Geometry: final body of the model. Coordinates: model frame, mm. Face numbers are marked on the shaded views. A direction names the side the tool comes from. Give positions to 0.01 mm unless a question says otherwise; leave off trailing zeros. Order: outer loops, then holes, each group sorted by start corner. A loop starts at its lowest first (then second) coordinate and runs counter-clockwise, first axis right, second up. Notation, with made-up numbers: (51, 79) -> (103, 79) arc R28 ccw to (103, 111) -> close; hole circle Ø4 at (-16.75, 45). An arc over 180 degrees is marked (long way). Answer in a Markdown table with one row per item. Add a question column.
Q1. Pull-direction query (Y, two-part tool) for the marked faces 1, 2 and 3; classes: +Y half, -Y half, draft (parallel to the pull), parting line (faces both ways), or undercut.
Q2. Contact query for flat-ended pins moving along their axis: P1, Ø6, axis at x = 14.5, z = 2, coming from the +Y side; P2, Ø1, axis at x = -7.5, y = 16, coming from the -Z side; P3, Ø10, axis at x = -19, z = -1.5, coming from the +Y side. Output: stop coordinate, or through.
Q3. Cut plane C-C on x = -10.5. Return the cut outline in (y, z).
Q4. Cut plane B-B on x = 0. Return the cut outline in (y, z), and give its area (3 significant figures).
Q5. Cut plane A-A on z = -10.5. Return the cut outline in (x, y).
Q6. Set-up query: the marked faces 4 and 5. Return all of +Z, -Z, +X, -X, +Y, -Y with unobstructed straight access to the full face (end or side cutting, diameter ignored); none if empty.
Q7. Cut plane D-D on y = 33. Return the cut outline in (x, z).
Q8. Line query: line 1 along Y through (x, z) = (0.5, -9.5); line 2 along X through (y, z) = (60, -4); line 3 along Y through (x, z) = (-3.5, -7.5). Output: solid intervals per line, ascending. Write a range as from..to.
from build123d import *

# Parameters (mm, degrees)
BOSS_EXTRUDE1_DEPTH = 6.35
SKETCH2_R           = 19.05
BOSS_EXTRUDE2_DEPTH = 25.4


with BuildPart() as part:
    # Sketch1 → Boss-Extrude1 (new body)
    with BuildSketch(Plane.XY):
        with BuildLine():
            ThreePointArc((38.1, 59.170454545), (0, 97.270454545), (-38.1, 59.170454545))
            ThreePointArc((-38.1, 59.170454545), (-24.166339939, 14.720454545), (-38.1, -29.729545455))
            ThreePointArc((-38.1, -29.729545455), (0, -67.829545455), (38.1, -29.729545455))
            ThreePointArc((38.1, -29.729545455), (24.166339939, 14.720454545), (38.1, 59.170454545))
        make_face()
    extrude(amount=BOSS_EXTRUDE1_DEPTH)

    # Sketch2 → Boss-Extrude2 (add)
    with BuildSketch(Plane(origin=(0, 0, 0), x_dir=(-1, 0, 0), z_dir=(0, 0, -1))):
        with Locations((0, 59.170454545)):
            Circle(SKETCH2_R)
        with Locations((0, -29.729545455)):
            Circle(SKETCH2_R)
    extrude(amount=BOSS_EXTRUDE2_DEPTH)


solid = part.part
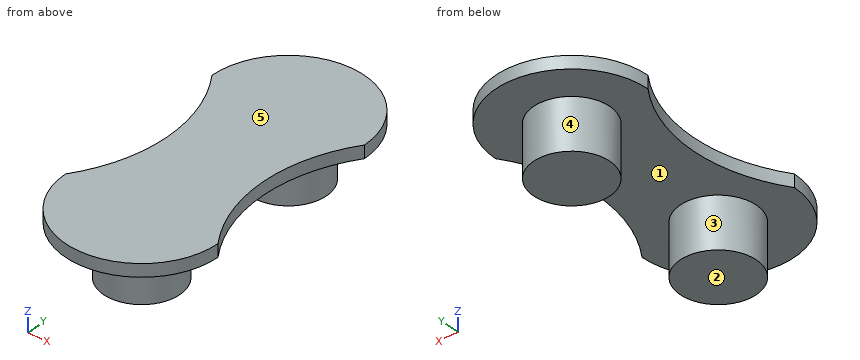
Completed:
| question | item | result |
|---|---|---|
| 1 | face 1 | undercut |
| 1 | face 2 | draft |
| 1 | face 3 | undercut |
| 2 | P1 | stops at y = 95.49 |
| 2 | P2 | stops at z = 0 |
| 2 | P3 | stops at y = 94.51 |
| 3 | outline | (-66.35, 0) -> (-45.62, 0) -> (-45.62, -25.4) -> (-13.83, -25.4) -> (-13.83, 0) -> (43.28, 0) -> (43.28, -25.4) -> (75.07, -25.4) -> (75.07, 0) -> (95.8, 0) -> (95.8, 6.35) -> (-66.35, 6.35) -> close |
| 4 | outline | (-67.83, 0) -> (-48.78, 0) -> (-48.78, -25.4) -> (-10.68, -25.4) -> (-10.68, 0) -> (40.12, 0) -> (40.12, -25.4) -> (78.22, -25.4) -> (78.22, 0) -> (97.27, 0) -> (97.27, 6.35) -> (-67.83, 6.35) -> close |
| 4 | area | 2,980 mm² |
| 5 | outline | circle Ø38.1 at (0, -29.73); circle Ø38.1 at (0, 59.17) |
| 6 | face 4 | -Z |
| 6 | face 5 | +Z, +X, -X, +Y, -Y |
| 7 | outline | (-26.34, 0) -> (26.34, 0) -> (26.34, 6.35) -> (-26.34, 6.35) -> close |
| 8 | line 1 | y = -48.77..-10.69, 40.13..78.21 |
| 8 | line 2 | x = -19.03..19.03 |
| 8 | line 3 | y = -48.46..-11, 40.44..77.9 |
